from build123d import *

# Parameters (mm, degrees)
SKETCH1_R                                 = 6.35
SKETCH1_R_2                               = 3.2639
SKETCH1_R_3                               = 1.099999959
INNER_SIDE_EXTRUDE_DEPTH                  = 2.032
OUTER_START                               = -9.525
SKETCH1_3_R                               = 7.14375
SKETCH1_3_R_2                             = 6.35
SKETCH1_3_R_3                             = 3.2639
SKETCH1_3_R_4                             = 1.099999959
OUTER_SIDE_EXTRUDE_DEPTH                  = 9.525
CLEVIS_PIN_CUT_DEPTH                      = 14.8849542
CLEVIS_PIN_CUT_DEPTH_BACK                 = 14.8849542
SKETCH2_R                                 = 1.63195
CHAMFER_SO_STEVE_DOESN_T_CUT_HIMSELF_SIZE = 0.396875


with BuildPart() as part:
    # Sketch1 → Inner Side Extrude (new body)
    with BuildSketch(Plane(origin=(0, 0, 0), x_dir=(0, 0, -1), z_dir=(1, 0, 0))):
        Circle(SKETCH1_R)
        Circle(SKETCH1_R_2, mode=Mode.SUBTRACT)
        with Locations((-5.06095, 0)):
            Circle(SKETCH1_R_3, mode=Mode.SUBTRACT)
        with Locations((5.06095, 0)):
            Circle(SKETCH1_R_3, mode=Mode.SUBTRACT)
    extrude(amount=INNER_SIDE_EXTRUDE_DEPTH)

    # Sketch1<3> → Outer Side Extrude (add)
    # profile 1 of 2: a face of its own
    with BuildSketch(Plane(origin=(0, 0, 0), x_dir=(0, 0, -1), z_dir=(1, 0, 0)).offset(OUTER_START)):
        Circle(SKETCH1_3_R)
        Circle(SKETCH1_3_R_2, mode=Mode.SUBTRACT)
    # profile 2 of 2: a face of its own
    with BuildSketch(Plane(origin=(0, 0, 0), x_dir=(0, 0, -1), z_dir=(1, 0, 0)).offset(OUTER_START)):
        Circle(SKETCH1_3_R_2)
        Circle(SKETCH1_3_R_3, mode=Mode.SUBTRACT)
        with Locations((-5.06095, 0)):
            Circle(SKETCH1_3_R_4, mode=Mode.SUBTRACT)
        with Locations((5.06095, 0)):
            Circle(SKETCH1_3_R_4, mode=Mode.SUBTRACT)
    extrude(amount=OUTER_SIDE_EXTRUDE_DEPTH)

    # Sketch2 → Clevis Pin Cut (cut, two sides: drawn at the far end of the back side and taken through both)
    with BuildSketch(Plane(origin=(0, 0, 0), x_dir=(1, 0, 0), z_dir=(0, 1, 0)).offset(-CLEVIS_PIN_CUT_DEPTH_BACK)):
        with Locations(Location((-4.7625, 0, 0), (0, 0, 270))):
            Circle(SKETCH2_R)
    extrude(amount=CLEVIS_PIN_CUT_DEPTH + CLEVIS_PIN_CUT_DEPTH_BACK, mode=Mode.SUBTRACT)

    # Chamfer so Steve Doesn't cut himself
    # the kernel refuses this chamfer: 0.396875 mm, written as the material it takes off along each edge
    with BuildSketch(Plane(origin=(2.032, 0, 0), x_dir=(0, 0, -1), z_dir=(0, -1, 0))) as chamfer_so_steve_doesn_t_cut_himself_piece_1:
        Polygon((3.2639 + CHAMFER_SO_STEVE_DOESN_T_CUT_HIMSELF_SIZE, 0), (3.2639, -CHAMFER_SO_STEVE_DOESN_T_CUT_HIMSELF_SIZE), (3.2639, 0), align=None)
    revolve(axis=Axis((2.032, 0, 0), (1, 0, 0)), mode=Mode.SUBTRACT)
    with BuildSketch(Plane(origin=(-9.525, 0, 0), x_dir=(0, 0, -1), z_dir=(0, -1, 0))) as chamfer_so_steve_doesn_t_cut_himself_piece_2:
        Polygon((7.14375, CHAMFER_SO_STEVE_DOESN_T_CUT_HIMSELF_SIZE), (7.14375 - CHAMFER_SO_STEVE_DOESN_T_CUT_HIMSELF_SIZE, 0), (7.14375, 0), align=None)
    revolve(axis=Axis((-9.525, 0, 0), (1, 0, 0)), mode=Mode.SUBTRACT)
    with BuildSketch(Plane(origin=(-9.525, 0, 0), x_dir=(0, 0, -1), z_dir=(0, -1, 0))) as chamfer_so_steve_doesn_t_cut_himself_piece_3:
        Polygon((3.2639, CHAMFER_SO_STEVE_DOESN_T_CUT_HIMSELF_SIZE), (3.2639 + CHAMFER_SO_STEVE_DOESN_T_CUT_HIMSELF_SIZE, 0), (3.2639, 0), align=None)
    revolve(axis=Axis((-9.525, 0, 0), (1, 0, 0)), mode=Mode.SUBTRACT)
    with BuildSketch(Plane(origin=(0, 0, 0), x_dir=(0, 0, -1), z_dir=(0, -1, 0))) as chamfer_so_steve_doesn_t_cut_himself_piece_4:
        Polygon((7.14375 - CHAMFER_SO_STEVE_DOESN_T_CUT_HIMSELF_SIZE, 0), (7.14375, -CHAMFER_SO_STEVE_DOESN_T_CUT_HIMSELF_SIZE), (7.14375, 0), align=None)
    revolve(axis=Axis((0, 0, 0), (1, 0, 0)), mode=Mode.SUBTRACT)
    with BuildSketch(Plane(origin=(2.032, 0, 0), x_dir=(0, 0, -1), z_dir=(0, -1, 0))) as chamfer_so_steve_doesn_t_cut_himself_piece_5:
        Polygon((6.35, -CHAMFER_SO_STEVE_DOESN_T_CUT_HIMSELF_SIZE), (6.35 - CHAMFER_SO_STEVE_DOESN_T_CUT_HIMSELF_SIZE, 0), (6.35, 0), align=None)
    revolve(axis=Axis((2.032, 0, 0), (1, 0, 0)), mode=Mode.SUBTRACT)


solid = part.part
Work out the finished part from the listing and answer in its coordinate system (mm). A direction names the side the tool comes from. Give positions to 0.01 mm unless a question says otherwise; leave off trailing zeros. Write each loop counter-clockwise with the first axis right and the second up, starting at its lowest first coordinate (ties: lowest second). Pieces come first, ordered by that corner, then holes. Notation, with made-up numbers: (76, 47.25) - (131, 47.25) arc R22 cw to (131, 84.25) - close; hole circle Ø5 at (84.5, -13). An arc over 180 degrees is marked (long way). One line per item, written item: value. Start each with the question number.
1. Find section C-C (x = -3.5). Write down the section's boundary in (y, z).
2. Given pin 1 (4 mm diameter, centred on y = 1.5, z = 0.5, fed in from +X); pin 2 (2.5 mm diameter, centred on x = -4.76, z = 0, fed in from +Y); pin 3 (4 mm diameter, centred on x = -8, y = 3.5, fed in from -Z), each flat-ended and moving along its own axis, determine where each tip first touches the part or whether it passes through.
3. For a pull along Z with two mould halves and no side action, classify faces 1 (the flat face through (0, -2.5, -6)), 2 (the cylindrical face through (-4.824, -6.338, -3.296)), 3 (the cylindrical face through (-3.827, -0.421, -6.077)) as +Z half, -Z half, draft (parallel to the pull), parting line (faces both ways), or undercut.
4. Consider probe 1 along Z at (x, y) = (-5.25, 0.25); probe 2 along Y at (x, z) = (-1.5, 0); probe 3 along Z at (x, y) = (-1, -2.25). Determine where each line is inside the solid, lowest interval first.
5. Find section B-B (z = 0). State how many separate pieces and enclosed holes the cut face has, then the cut area to 3 significant figures.
6. Find section A-A (y = 0). Write down the section's boundary in (x, z) (3 decimals), then the cut area to 3 significant figures.
7. Find section D-D (x = -1). Write down the section's boundary in (y, z).
8. For faces 4 (the cylindrical face through (0.81, -6.2, 1.38)), 5 (the cylindrical face through (-3.822, 2.752, -1.755)), determine the directions among +Z, -Z, +X, -X, +Y, -Y from which every point of the face is accessible in a straight line to the end or side of a thin tool.
Geometry results:
1. outline: (-7.07, -1.03) arc R7.14 ccw to (7.07, -1.03) - (3.1, -1.03) arc R3.26 cw to (-3.1, -1.03) - close; (-7.07, 1.03) - (-3.1, 1.03) arc R3.26 cw to (3.1, 1.03) - (7.07, 1.03) arc R7.14 ccw to start; hole circle Ø2.2 at (0, -5.06); hole circle Ø2.2 at (0, 5.06)
2. pin 1: x = 1.95
2. pin 2: through
2. pin 3: z = -6.98
3. face 1: draft
3. face 2: parting line
3. face 3: undercut
4. probe 1: -7.14 to -6.13, -3.99 to -3.25, 3.25 to 3.99, 6.13 to 7.14
4. probe 2: -7.14 to -3.26, 3.26 to 7.14
4. probe 3: -6.78 to -2.36, 2.36 to 6.78
5. separate pieces: 4
5. enclosed holes: 0
5. area: 60.3 mm2
6. outline: (-9.525, -6.747) - (-9.128, -7.144) - (-0.397, -7.144) - (0, -6.747) - (0, -6.35) - (1.635, -6.35) - (1.824, -6.161) - (-9.525, -6.161) - close; (-9.525, -3.961) - (2.032, -3.961) - (2.032, -3.661) - (1.635, -3.264) - (-9.128, -3.264) - (-9.525, -3.661) - close; (-9.525, 3.661) - (-9.128, 3.264) - (1.635, 3.264) - (2.032, 3.661) - (2.032, 3.961) - (-9.525, 3.961) - close; (-9.525, 6.161) - (1.824, 6.161) - (1.635, 6.35) - (0, 6.35) - (0, 6.747) - (-0.397, 7.144) - (-9.128, 7.144) - (-9.525, 6.747) - close
6. area: 34.9 mm2
7. outline: circle Ø14.29 at (0, 0); hole circle Ø6.53 at (0, 0); hole circle Ø2.2 at (0, -5.06); hole circle Ø2.2 at (0, 5.06)
8. face 4: +X
8. face 5: +X, -X
